Geometry: see drawing. Coordinates: mm, zero at the bounding-box minimum. A direction names the side the tool comes from. Coordinates: 2 decimals unless noted, no trailing zeros. Order: outer loops, then holes, each group sorted by start corner. A loop starts at its lowest first (then second) coordinate and runs counter-clockwise, first axis right, second up. Notation, with made-up numbers: (46, 44.5) -> (102, 44.5) arc R19 cw to (102, 62.5) -> close; hole circle Ø9 at (89, 7.5). An arc over 180 degrees is marked (long way). One line per item, written item: value. Start each with the question number.
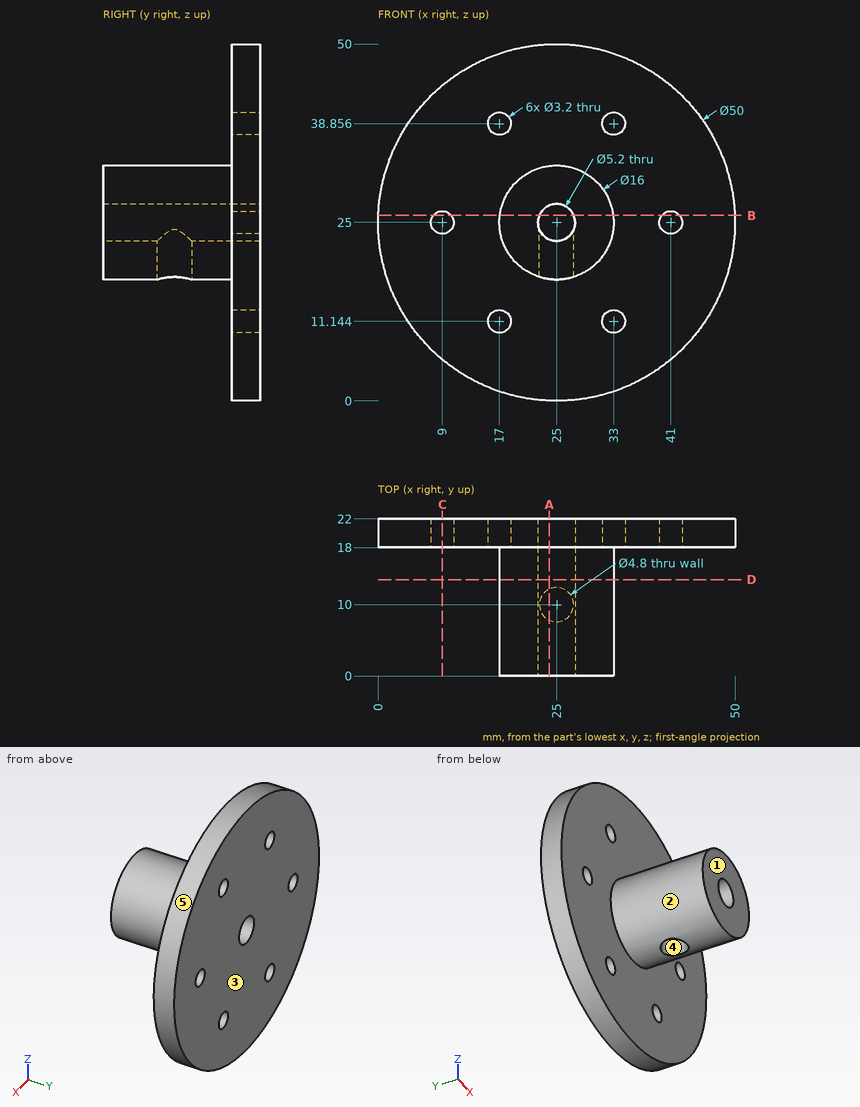
1) Section query C-C, the plane x = 9. Return the cut outline in (y, z), plus the area to 3 significant figures.
2) Section query D-D, the plane y = 13.5. Return the cut outline in (x, z), plus the area to 3 significant figures.
3) Section query B-B, the plane z = 26. Return the cut outline in (x, y).
4) Ray query, line 1 along Z through (x, y) = (25, 13.75); line 2 along Y through (x, z) = (6.5, 26). Return the intervals inside material, ascending. Write a range as from..to.
5) Section query A-A, the plane x = 24. Return the cut outline in (y, z).
6) Pin query (flat end, axial travel): pin 1 Ø3 at (x, z) = (25, 25) entering from -Y; pin 2 Ø3.5 at (x, z) = (17, 38.86) entering from -Y; pin 3 Ø10 at (y, z) = (13.5, 20.5) entering from -X; pin 4 Ø10 at (y, z) = (18.5, 43.5) entering from +X. Return the tip coordinate at first contact, or that it passes through.
7) Mould query, pull axis X, two halves, no side actions, for the marked faces 3, 4 and 5. Classes: +X half, -X half, draft (parallel to the pull), parting line (faces both ways), or undercut.
8) Access query for the marked faces 1 and 2. Directions: +Z, -Z, +X, -X, +Y, -Y. A direction counts if a zero-diameter tool reaches every point of the face in a straight line with its end or side. Return the directions, or none.
Entries:
1. outline: (18, 5.79) -> (22, 5.79) -> (22, 23.4) -> (18, 23.4) -> close; (18, 26.6) -> (22, 26.6) -> (22, 44.21) -> (18, 44.21) -> close
1. area: 141 mm2
2. outline: circle Ø16 at (25, 25); hole circle Ø5.2 at (25, 25)
2. area: 180 mm2
3. outline: (0.02, 18) -> (7.75, 18) -> (7.75, 22) -> (0.02, 22) -> close; (10.25, 18) -> (17.06, 18) -> (17.06, 0) -> (22.6, 0) -> (22.6, 22) -> (10.25, 22) -> close; (27.4, 0) -> (32.94, 0) -> (32.94, 18) -> (39.75, 18) -> (39.75, 22) -> (27.4, 22) -> close; (42.25, 18) -> (49.98, 18) -> (49.98, 22) -> (42.25, 22) -> close
4. line 1: z = 17..22.4, 27.6..33
4. line 2: y = 18..22
5. outline: (0, 17.06) -> (7.82, 17.06) -> (7.82, 22.6) -> (0, 22.6) -> close; (0, 27.4) -> (22, 27.4) -> (22, 49.98) -> (18, 49.98) -> (18, 32.94) -> (0, 32.94) -> close; (12.18, 17.06) -> (18, 17.06) -> (18, 0.02) -> (22, 0.02) -> (22, 22.6) -> (12.18, 22.6) -> close
6. pin 1: passes through
6. pin 2: stops at y = 18
6. pin 3: stops at x = 0.11
6. pin 4: stops at x = 46.04
7. face 3: draft
7. face 4: undercut
7. face 5: parting line
8. face 1: +Z, -Z, +X, -X, -Y
8. face 2: -Y
